Verification items for this drawing (mm, ordinates from the low corner). Round coordinates to 2 decimals unless told otherwise and drop trailing zeros. Loops run counter-clockwise (first coordinate to the right, second up) from the corner with the lowest first, then second, coordinate; pieces in that order, holes last. Notation, with made-up numbers: (26, 65) - (57, 65) arc R10 ccw to (57, 79) - close; hole circle Ø7 at (-29, 47.5). An arc over 180 degrees is marked (long way). Answer in a Markdown table with one row per item. Add a question column.
(1) Cross-section at B-B on y = 18. Enter the section's corners in (x, z).
(2) Mould release check, pull along Y, two halves, no side actions. Record for the marked faces 1, 2 and 3: +Y half, -Y half, draft (parallel to the pull), parting line (faces both ways), or undercut.
(3) Gauge pin test, flat ends, axial feed: pin 1 (4 mm diameter, centred on x = 28, z = 3.5, fed in from -Y); pin 2 (3 mm diameter, centred on x = 4.5, y = 4, fed in from +Z). Record the tip position at first contact, or that the pin passes through.
(4) Cross-section at A-A on z = 10.5. Enter the section's corners in (x, y).
(5) Thickness scan on line 1 along Y through (x, z) = (8.5, 31.5); line 2 along X through (y, z) = (14, 28.5). Record the ranges inside material, lowest first.
(6) Cross-section at C-C on x = 21.5. Enter the section's corners in (y, z).
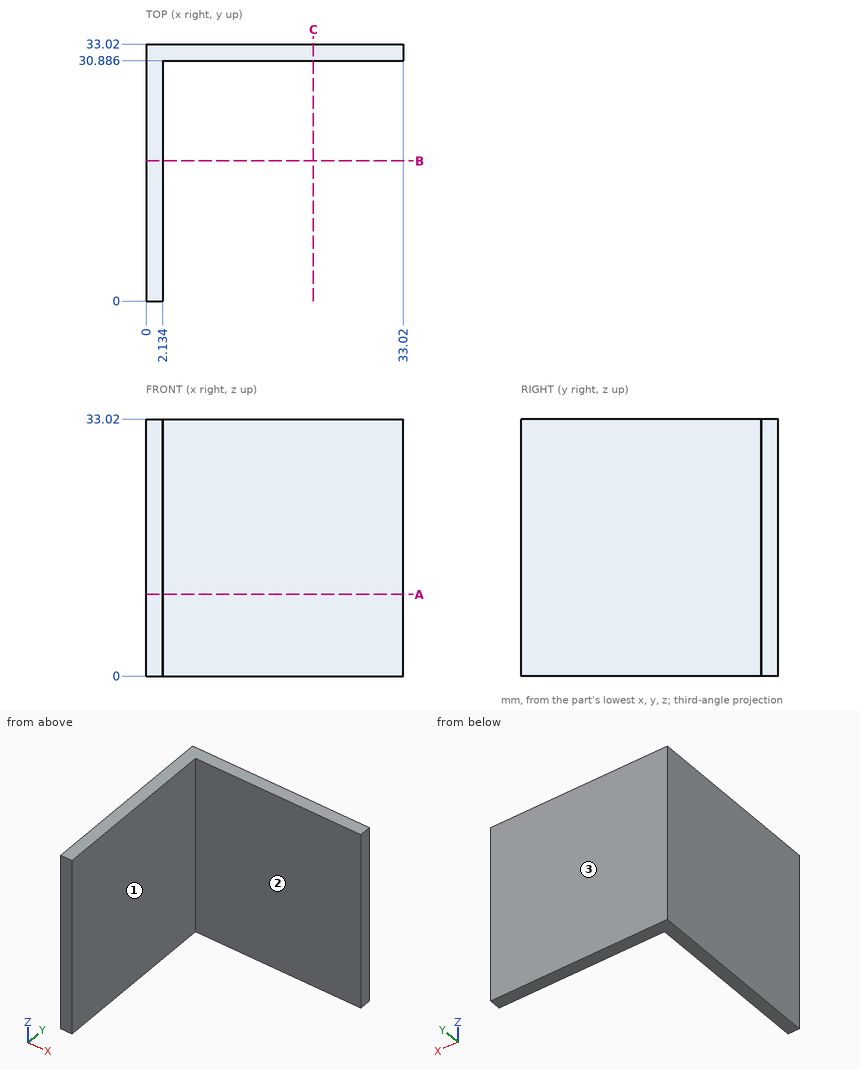
Answers:
| question | item | result |
|---|---|---|
| 1 | outline | (0, 0) - (2.13, 0) - (2.13, 33.02) - (0, 33.02) - close |
| 2 | face 1 | draft |
| 2 | face 2 | -Y half |
| 2 | face 3 | +Y half |
| 3 | pin 1 | stops at y = 30.89 |
| 3 | pin 2 | passes through |
| 4 | outline | (0, 0) - (2.13, 0) - (2.13, 30.89) - (33.02, 30.89) - (33.02, 33.02) - (0, 33.02) - close |
| 5 | line 1 | y = 30.89 to 33.02 |
| 5 | line 2 | x = 0 to 2.13 |
| 6 | outline | (30.89, 0) - (33.02, 0) - (33.02, 33.02) - (30.89, 33.02) - close |
